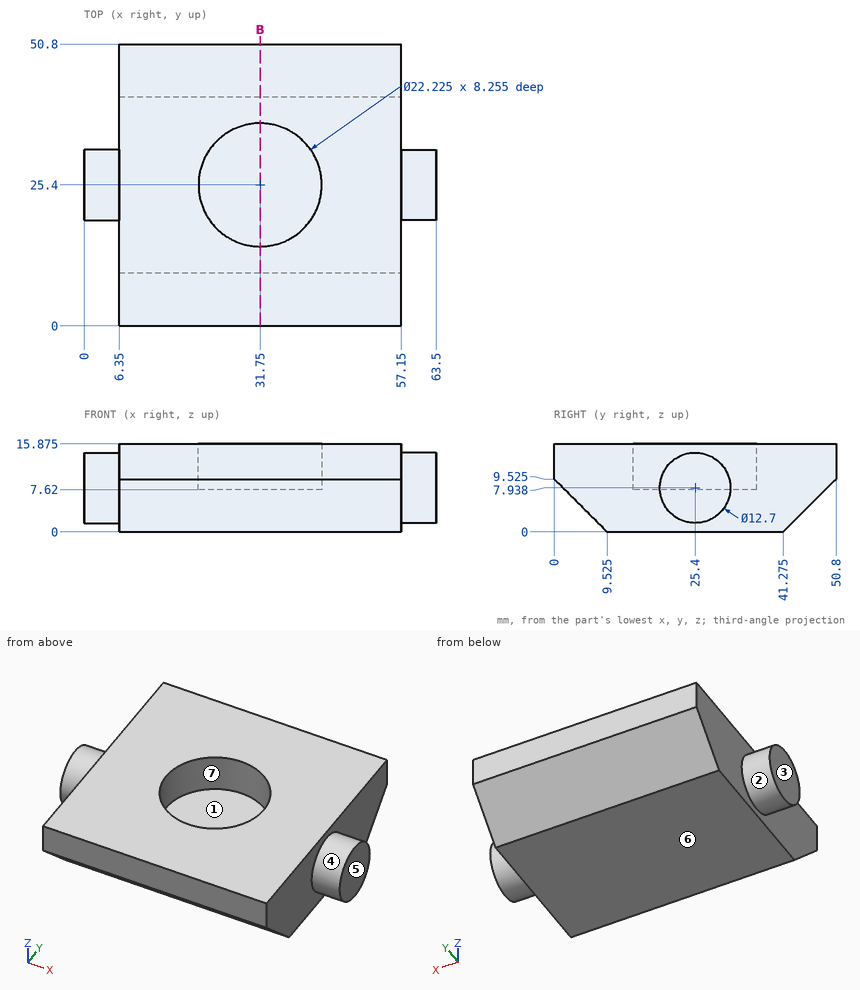
Source: three-view drawing plus pictorial views. Frame: mm from the lowest corner of the part. A direction names the side the tool comes from. Round coordinates to 2 decimals unless told otherwise and drop trailing zeros. Loops run counter-clockwise (first coordinate to the right, second up) from the corner with the lowest first, then second, coordinate; pieces in that order, holes last.
Q1. Ray query, line 1 (X direction, y = 25.5, z = 14.75); line 2 (Y direction, x = 31.75, z = 12.25); line 3 (X direction, y = 10, z = 5.75). Return the intervals inside material, ascending.
Q2. Section B-B, the plane x = 31.75. Return loops of the section in (y, z) (1 decimal).
Q3. Access query for the marked faces 1, 2, 3 and 4. Directions: +Z, -Z, +X, -X, +Y, -Y. A direction counts if a zero-diameter tool reaches every point of the face in a straight line with its end or side. Return the directions, or none.
Q4. First-contact query: P1, Ø1.5, axis at x = 14.5, z = 4.5, coming from the +Y side (1 decimal); P2, Ø1.5, axis at y = 24.5, z = 9.5, coming from the -X side; P3, Ø8, axis at y = 45.5, z = 13.5, coming from the -X side. Flat tips, straight axial feed; report the tip coordinate or a pass-through.
Q5. Mould query, pull axis X, two halves, no side actions, for the marked faces 5, 6 and 7. Classes: pulls with the +X half, pulls with the -X half, needs draft (parallel to the pull), parting line crosses it, or undercut.
Solutions:
1. line 1: x = 6.35 to 20.64, 42.86 to 57.15
1. line 2: y = 0 to 14.29, 36.51 to 50.8
1. line 3: x = 6.35 to 57.15
2. outline: (0, 9.5) - (9.5, 0) - (41.3, 0) - (50.8, 9.5) - (50.8, 15.9) - (36.5, 15.9) - (36.5, 7.6) - (14.3, 7.6) - (14.3, 15.9) - (0, 15.9) - close
3. face 1: +Z
3. face 2: -X
3. face 3: +Z, -Z, -X, +Y, -Y
3. face 4: +X
4. P1: stops at y = 46.5
4. P2: stops at x = 0
4. P3: stops at x = 6.35
5. face 5: pulls with the +X half
5. face 6: needs draft
5. face 7: undercut
